Check sheet for the modelled part. Datum: model origin and axes. Units: mm. A direction names the side the tool comes from. Give positions to 0.01 mm unless a question says otherwise; leave off trailing zeros. Write each loop counter-clockwise with the first axis right and the second up, starting at its lowest first coordinate (ties: lowest second). Pieces come first, ordered by that corner, then holes. Notation, with made-up numbers: M 29.5,79.25 L 45.5,79.25 A11 ccw 45.5,87.25 Z; hole C 27,-24 d10. An arc over 180 degrees is marked long. Use CSV: the item, a comma, the result in double quotes. Start each with the question number.
1. Depth check by flat-ended pin: P1, Ø8, axis at y = 38, z = 13, coming from the -X side; P2, Ø0.8, axis at x = -9.5, y = 29.5, coming from the -Z side; P3, Ø4, axis at y = 11.5, z = 12, coming from the +X side. Enter the tip coordinate at first touch or a pass-through.
2. Cross-section at C-C, the plane z = 0. Enter the section's corners in (x, y) (3 decimals).
3. Access from +Z, -Z, +X, -X, +Y, -Y to the whole of each face (thin tool, end or side, straight path). Record for faces 5 (the face through (15.748, 32.239, -4.959)), 6 (the face through (-10, 35, -11)), 7 (the face through (-4, 58, -14)).
4. Mould release check, pull along Z, two halves, no side actions. Record for faces 1 (the face through (0, 59.92, -15)), 2 (the face through (-9, 35, -10.319)), 3 (the face through (-0.448, 35.414, 12.692)), 4 (the face through (0, 68, 19.05)): +Z half, -Z half, draft (parallel to the pull), parting line (faces both ways), or undercut.
5. Cross-section at B-B, the plane x = 0. Enter the section's corners in (y, z) (3 decimals), and give its area (3 significant figures).
6. Scan lines: line 1 (Z direction, x = 0, y = 40); line 2 (Z direction, x = -8, y = 61.5); line 3 (Y direction, x = 4.5, z = 11.5) (3 decimals). Record each from-to range of solid material in increasing order.
7. Cross-section at D-D, the plane x = 15.5. Enter the section's corners in (y, z) (3 decimals).
8. Cross-section at A-A, the plane y = 12.5. Enter the section's corners in (x, z).
Autodesk Inventor part; units mm, degrees
ref_plane "YZ Plane" through (0, 0, 0) normal (1, 0, 0) x (0, 1, 0)
ref_plane "XZ Plane" through (0, 0, 0) normal (0, 1, 0) x (-1, 0, 0)
ref_plane "XY Plane" through (0, 0, 0) normal (0, 0, 1) x (1, 0, 0)
sketch "Sketch1" plane through (0, 0, 0) normal (0, 1, 0) x (-1, 0, 0)
  line L0 (31.75, -31.75) -> (-31.75, -31.75)
  line L1 (-31.75, -31.75) -> (-31.75, 31.75)
  line L2 (-31.75, 31.75) -> (31.75, 31.75)
  line L3 (31.75, 31.75) -> (31.75, -31.75)
  point P0 (0, 0)
  point P1 (-31.75, 0)
  point P2 (0, -31.75)
  dimension "d0" = 63.5
  dimension "d1" = 63.5
extrude "Extrusion1" add sketch "Sketch1" along normal blind 69.85
sketch "Sketch2" plane through (0, 69.85, 0) normal (0, 1, 0) x (1, 0, 0)
  circle A0 centre (0, 0) radius 12.7
  line L0 (-10, 12.7) -> (10, 12.7)
  line L1 (10, 12.7) -> (10, 10.3187)
  line L2 (10, 10.3187) -> (-10, 10.3187)
  line L3 (-10, 10.3187) -> (-10, 12.7)
  point P0 (-12.7, 0)
  point P1 (12.7, 0)
  point P2 (0, 12.7)
  point P3 (-7.4036, 10.3187)
  point P4 (0, 7.5)
  point P5 (7.4036, 10.3187)
  dimension "d4" = 25.4
  dimension "d7" = 20
  dimension "d8" = 2.3813
extrude "Extrusion2" cut sketch "Sketch2" against normal through all
sketch "Sketch4" plane through (0, 69.85, 0) normal (0, 1, 0) x (1, 0, 0)
  circle A0 centre (0, 0) radius 16.51
  line L0 (-23.2494, 25.4) -> (-10.5494, 25.4)
  line L1 (-10.5494, 25.4) -> (-10.5494, 12.7)
  line L2 (-10.5494, 12.7) -> (-23.2494, 12.7)
  line L3 (-23.2494, 12.7) -> (-23.2494, 25.4)
  line L4 (-31.75, 31.75) -> (-31.75, -31.75)
  line L5 (-31.75, 0) -> (31.75, 0)
  line L6 (10.5494, 25.4) -> (23.2494, 25.4)
  line L7 (23.2494, 25.4) -> (23.2494, 12.7)
  line L8 (23.2494, 12.7) -> (10.5494, 12.7)
  line L9 (10.5494, 12.7) -> (10.5494, 25.4)
  line L10 (10.5494, -12.7) -> (23.2494, -12.7)
  line L11 (23.2494, -12.7) -> (23.2494, -25.4)
  line L12 (23.2494, -25.4) -> (10.5494, -25.4)
  line L13 (10.5494, -25.4) -> (10.5494, -12.7)
  line L14 (-23.2494, -12.7) -> (-10.5494, -12.7)
  line L15 (-10.5494, -12.7) -> (-10.5494, -25.4)
  line L16 (-10.5494, -25.4) -> (-23.2494, -25.4)
  line L17 (-23.2494, -25.4) -> (-23.2494, -12.7)
  line L18 (-23.2494, 25.4) -> (23.2494, 25.4)
  line L19 (23.2494, 25.4) -> (23.2494, -25.4)
  line L20 (23.2494, -25.4) -> (-23.2494, -25.4)
  line L21 (-23.2494, -25.4) -> (-23.2494, 25.4)
  line L22 (31.75, -31.75) -> (31.75, 31.75)
  line L23 (-31.75, 31.75) -> (31.75, 31.75)
  line L24 (31.75, 31.75) -> (31.75, -31.75)
  line L25 (31.75, -31.75) -> (-31.75, -31.75)
  line L26 (-31.75, -31.75) -> (-31.75, 31.75)
  dimension "d10" = 33.02
  dimension "d11" = 12.7
  dimension "d12" = 12.7
  dimension "d13" = 12.7
  dimension "d14" = 12.7
  dimension "d15" = 12.7
  dimension "d16" = 12.7
  dimension "d17" = 12.7
  dimension "d18" = 12.7
  dimension "d19" = 12.7
  dimension "d20" = 12.7
  dimension "d21" = 12.7
  dimension "d22" = 12.7
sketch "Sketch5" plane through (0, 69.85, 0) normal (0, 1, 0) x (1, 0, 0)
  point P0 (0, 0)
extrude "Extrusion3" cut sketch "Sketch4" against normal blind 50.8 contours L19 L7 L6 L18 L0 L3 L21 L5 L4 L23 L22 | L5 L22 L25 L4 L21 L17 L16 L20 L12 L11 L19
sketch "Sketch6" plane through (0, 69.85, 0) normal (0, 1, 0) x (1, 0, 0)
  point P0 (0, 0)
sketch "Sketch7" plane through (0, 0, 0) normal (0, -1, 0) x (1, 0, 0)
  circle A0 centre (0, 0) radius 16.51
  line L0 (-23.2494, 25.4) -> (23.2494, 25.4)
  line L1 (23.2494, 25.4) -> (23.2494, -25.4)
  line L2 (-23.2494, 25.4) -> (23.2494, 25.4)
  line L3 (23.2494, 25.4) -> (23.2494, -25.4)
  line L4 (23.2494, -25.4) -> (-23.2494, -25.4)
  line L5 (-23.2494, -25.4) -> (-23.2494, 25.4)
  dimension "d25" = 33.02
extrude "Extrusion4" cut sketch "Sketch7" against normal blind 66.675
sketch "Sketch9" plane through (0, 69.85, 0) normal (0, 1, 0) x (1, 0, 0)
  line L0 (-19.05, 19.05) -> (19.05, 19.05)
  line L1 (19.05, 19.05) -> (19.05, -19.05)
  line L2 (19.05, -19.05) -> (-19.05, -19.05)
  line L3 (-19.05, -19.05) -> (-19.05, 19.05)
  line L4 (23.2494, -25.4) -> (23.2494, 25.4)
  line L5 (-23.2494, 25.4) -> (23.2494, 25.4)
  line L6 (23.2494, 25.4) -> (23.2494, -25.4)
  line L7 (23.2494, -25.4) -> (-23.2494, -25.4)
  line L8 (-23.2494, -25.4) -> (-23.2494, 25.4)
  line L9 (31.75, -31.75) -> (-31.75, -31.75)
  line L10 (-31.75, -31.75) -> (-31.75, 31.75)
  line L11 (31.75, -31.75) -> (-31.75, -31.75)
  line L12 (-31.75, -31.75) -> (-31.75, 31.75)
  line L13 (-31.75, 31.75) -> (31.75, 31.75)
  line L14 (31.75, 31.75) -> (31.75, -31.75)
  point P0 (0, 0)
  point P1 (0, 19.05)
  point P2 (19.05, 0)
  point P3 (23.2494, 25.4)
  dimension "d42" = 38.1
  dimension "d43" = 38.1
extrude "Extrusion6" cut sketch "Sketch9" against normal through all contours L7 L8 L5 L4 | L9 L10 L13 L14
sketch "Sketch21" plane through (0, 0, 0) normal (0, -1, 0) x (1, 0, 0)
  arc A0 (7.4036, -10.3187) -> (-7.4036, -10.3187) centre (0, 0) ccw
  circle A1 centre (0, 0) radius 16.51
extrude "Extrusion15" add sketch "Sketch21" along normal blind 3.175
sketch "Sketch22" plane through (-10, 69.85, -12.7) normal (0, 0, 1) x (1, 0, 0)
  line L0 (20, -69.85) -> (0, -69.85)
  line L1 (6, -12.93) -> (14, -12.93)
  line L2 (14, -12.93) -> (14, -9.93)
  line L3 (14, -9.93) -> (6, -9.93)
  line L4 (6, -9.93) -> (6, -12.93)
  line L5 (29.05, 0) -> (-9.05, 0)
  point P0 (10, -69.85)
  point P1 (10, -11.43)
  point P2 (14, -11.43)
  point P3 (10, -9.93)
  dimension "d87" = 58.42
  dimension "d88" = 8
  dimension "d89" = 3
  dimension "d92" = 11.43
extrude "Extrusion16" cut sketch "Sketch22" against normal blind 6.35
properties part number "WaterCollector_3DPrint"
Worked answers:
1,P1,"stops at x = -13.84"
1,P2,"stops at z = -13.78"
1,P3,"stops at x = 13.14"
2,outline,"M -19.05,66.675 L -16.51,66.675 L -16.51,-3.175 L 16.51,-3.175 L 16.51,66.675 L 19.05,66.675 L 19.05,69.85 L 12.7,69.85 L 12.7,0 L -12.7,0 L -12.7,69.85 L -19.05,69.85 Z"
3,face 5,"-Y"
3,face 6,"+Y"
3,face 7,"-Z"
4,face 1,"draft"
4,face 2,"undercut"
4,face 3,"undercut"
4,face 4,"+Z half"
5,outline,"M -3.175,-16.51 L 56.92,-16.51 L 56.92,-12.7 L 0,-12.7 L 0,12.7 L 69.85,12.7 L 69.85,19.05 L 66.675,19.05 L 66.675,16.51 L -3.175,16.51 Z; M 59.92,-16.51 L 66.675,-16.51 L 66.675,-19.05 L 69.85,-19.05 L 69.85,-12.7 L 59.92,-12.7 Z"
5,area,"642 mm^2"
6,line 1,"z = -16.51 to -12.7, 12.7 to 16.51"
6,line 2,"z = -14.44 to -12.7, -10.32 to -9.86, 9.86 to 14.44"
6,line 3,"y = -3.175 to 0"
7,outline,"M -3.175,-5.686 L 66.675,-5.686 L 66.675,-19.05 L 69.85,-19.05 L 69.85,19.05 L 66.675,19.05 L 66.675,5.686 L -3.175,5.686 Z"
8,outline,"C 0,0 d33.02; hole M -10,-12.7 L 10,-12.7 L 10,-10.32 L 7.4,-10.32 A12.7 ccw long -7.4,-10.32 L -10,-10.32 Z"
